Check sheet for the modelled part. Datum: model origin and axes. Units: mm. Face numbers are marked on the shaded views. A direction names the side the tool comes from. Give positions to 0.01 mm unless a question says otherwise; leave off trailing zeros. Order: outer loops, then holes, each group sorted by start corner. A loop starts at its lowest first (then second) coordinate and runs counter-clockwise, first axis right, second up. Notation, with made-up numbers: (37, -35) -> (61, -35) arc R33 ccw to (61, 1) -> close; hole circle Ø11 at (30, -2.5). An arc over 180 degrees is marked (long way). One line per question, with ' | ' between items. Start each with the question number.
from build123d import *

# Parameters (mm, degrees)
TABAN_FLAN_1_DEPTH    = 15
KES_EKSTR_ZYON1_DEPTH = 101.124921973


# Sheet-metal steps are written as plain solids
with BuildPart() as part:
    # Çizim1 → Taban-Flanş1 (new body)
    with BuildSketch(Plane.XY):
        with BuildLine():
            ThreePointArc((-70, 0), (-68.290514437, -15.375488216), (-63.245553203, -30))
            ThreePointArc((-63.245553203, -30), (-37.049172752, -49.441795719), (-5, -55.531483348))
            ThreePointArc((-5, -55.531483348), (2.861742557, -60.912841793), (0, -70))
            ThreePointArc((0, -70), (15.375488216, -68.290514437), (30, -63.245553203))
            ThreePointArc((30, -63.245553203), (49.441795719, -37.049172752), (55.531483348, -5))
            ThreePointArc((55.531483348, -5), (60.912841793, 2.861742557), (70, 0))
            ThreePointArc((70, 0), (68.290514437, 15.375488216), (63.245553203, 30))
            ThreePointArc((63.245553203, 30), (37.049172752, 49.441795719), (5, 55.531483348))
            ThreePointArc((5, 55.531483348), (-2.861742557, 60.912841793), (0, 70))
            ThreePointArc((0, 70), (-15.375488216, 68.290514437), (-30, 63.245553203))
            ThreePointArc((-30, 63.245553203), (-49.441795719, 37.049172752), (-55.531483348, 5))
            ThreePointArc((-55.531483348, 5), (-60.912841793, -2.861742557), (-70, 0))
        make_face()
    extrude(amount=-TABAN_FLAN_1_DEPTH)

    # Çizim8 → Kes-Ekstrüzyon1 (cut, through all)
    with BuildSketch(Plane.XY):
        with BuildLine():
            Line((-15.451192956, -8.216485638), (-14.507693087, 9.786564326))
            ThreePointArc((-14.507693087, 9.786564326), (0.915879234, 17.476016858), (15.451192956, 8.216485638))
            Line((15.451192956, 8.216485638), (14.507693087, -9.786564326))
            ThreePointArc((14.507693087, -9.786564326), (-0.915879234, -17.476016858), (-15.451192956, -8.216485638))
        make_face()
    extrude(amount=-KES_EKSTR_ZYON1_DEPTH, mode=Mode.SUBTRACT)


solid = part.part
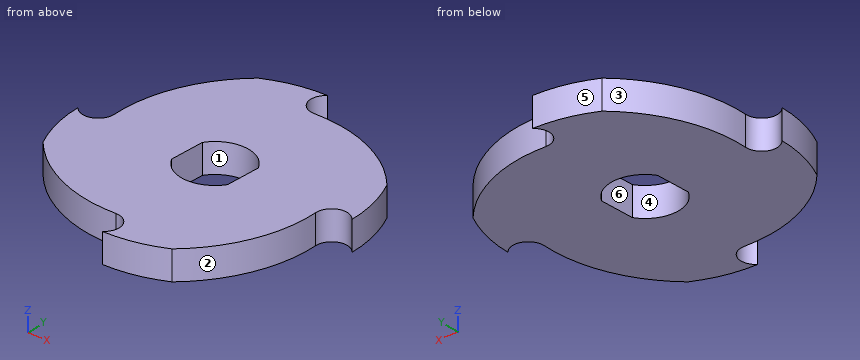
1. Cross-section at A-A on x = -8.5. Record the boundary of the cut face in (y, z).
2. Cross-section at B-B on z = -7. Record the boundary of the cut face in (x, y).
3. Go/stop test with flat-tipped pins: pin 1 (1 mm diameter, centred on x = 51.5, z = -12, fed in from +Y); pin 2 (4 mm diameter, centred on x = 32, z = -3.5, fed in from +Y); pin 3 (3 mm diameter, centred on y = -17, z = -2.5, fed in from +X). Record where each tip stops, or that it passes through.
4. Cross-section at C-C on y = 46.5. Record the boundary of the cut face in (x, z).
5. Mould release check, pull along X, two halves, no side actions. Record for the marked faces 1, 2, 3 and 4: +X half, -X half, draft (parallel to the pull), parting line (faces both ways), or undercut.
6. Scan lines: probe 1 along Y at (x, z) = (-10, -11.5); probe 2 along Y at (x, z) = (-24.5, -9); probe 3 along X at (y, z) = (48, -11.75). Record each from-to range of solid material in increasing order.
7. Tool access check on the marked faces 5 and 6. Record the directions out of +Z, -Z, +X, -X, +Y, -Y that give a thin tool (end or side, any length) a straight path to the whole face; none if there is none.
8. Cross-section at D-D on x = -47. Record the boundary of the cut face in (y, z), and give its area (3 significant figures).
Response values:
1) outline: (-55.58, -15) -> (-15.3, -15) -> (-15.3, 0) -> (-55.58, 0) -> close; (15.3, -15) -> (69.48, -15) -> (69.48, 0) -> (15.3, 0) -> close
2) outline: (-70, 0) arc R70 ccw to (-63.25, -30) arc R73 ccw to (-5, -55.53) arc R8 cw to (0, -70) arc R70 ccw to (30, -63.25) arc R73 ccw to (55.53, -5) arc R8 cw to (70, 0) arc R70 ccw to (63.25, 30) arc R73 ccw to (5, 55.53) arc R8 cw to (0, 70) arc R70 ccw to (-30, 63.25) arc R73 ccw to (-55.53, 5) arc R8 cw to start; hole (-15.45, -8.22) arc R17.5 ccw to (14.51, -9.79) -> (15.45, 8.22) arc R17.5 ccw to (-14.51, 9.79) -> close
3) pin 1: stops at y = 41.39 | pin 2: stops at y = 52.11 | pin 3: stops at x = 55.17
4) outline: (-44.44, -15) -> (43.01, -15) -> (43.01, 0) -> (-44.44, 0) -> close
5) face 1: undercut | face 2: +X half | face 3: -X half | face 4: undercut
6) probe 1: y = -55.55 to -14.36, 14.36 to 69.28 | probe 2: y = -53.63 to 65.57 | probe 3: x = -43.48 to 40.14
7) face 5: +Z, -Z, -X, +Y | face 6: +Z, -Z
8) outline: (-44.13, -15) -> (42.09, -15) -> (42.09, 0) -> (-44.13, 0) -> close | area: 1,290 mm²
